Check sheet for the modelled part. Datum: model origin and axes. Units: mm. Face numbers are marked on the shaded views. A direction names the side the tool comes from. Coordinates: 2 decimals unless noted, no trailing zeros. Loops run counter-clockwise (first coordinate to the right, second up) from the corner with the lowest first, then second, coordinate; pieces in that order, holes last. Notation, with made-up numbers: M 49.5,35 L 80.5,35 A11 ccw 80.5,44 Z; hole C 83.5,47.5 d11. An arc over 180 degrees is marked long. Return JSON: item names as keys, results as strings.
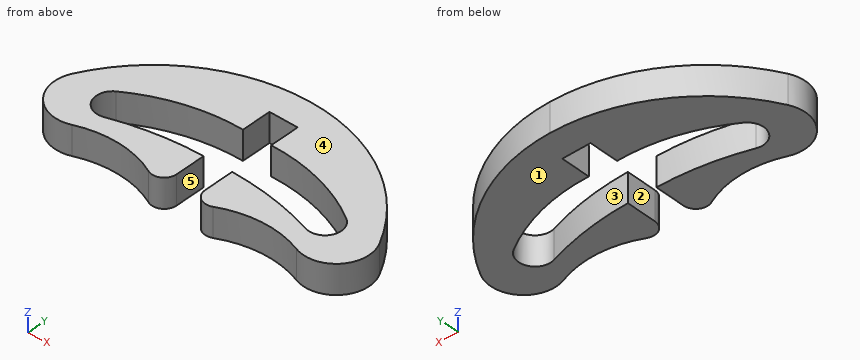
from build123d import *

# Parameters (mm, degrees)
EXTRUDE_1_DEPTH     = 3
SKETCH_2_W          = 2.925
SKETCH_2_H          = 8.058162309
CUT_EXTRUDE_1_DEPTH = 3
FILLET_1_R          = 1.27


with BuildPart() as part:
    # 스케치1 → 보스-돌출1 (new body)
    with BuildSketch(Plane.XY):
        with BuildLine():
            Line((-1.4475, 2.128), (-1.4475, 5.128))
            Line((-1.4475, 5.128), (1.4475, 5.128))
            Line((1.4475, 5.128), (1.4475, 2.128))
            ThreePointArc((1.4475, 2.128), (6.843352857, 1.44491364), (11.796869597, -0.801084345))
            ThreePointArc((11.796869597, -0.801084345), (12.394248626, -2.935784128), (10.351605925, -3.7968391))
            ThreePointArc((10.351605925, -3.7968391), (5.891355798, -2.693189603), (1.311601441, -2.322078509))
            Line((1.311601441, -2.322078509), (1.311601441, -7.845124291))
            ThreePointArc((1.311601441, -7.845124291), (6.16890602, -5.580674334), (11.498183086, -6.146313204))
            ThreePointArc((11.498183086, -6.146313204), (15.270849943, -5.260819217), (15.756720066, -1.416206748))
            ThreePointArc((15.756720066, -1.416206748), (9.210946066, 5.555889316), (0, 8.128))
            ThreePointArc((0, 8.128), (-9.210946066, 5.555889316), (-15.756720066, -1.416206748))
            ThreePointArc((-15.756720066, -1.416206748), (-15.270849943, -5.260819217), (-11.498183086, -6.146313204))
            ThreePointArc((-11.498183086, -6.146313204), (-6.16890602, -5.580674334), (-1.311601441, -7.845124291))
            Line((-1.311601441, -7.845124291), (-1.311601441, -2.322078509))
            ThreePointArc((-1.311601441, -2.322078509), (-5.891355798, -2.693189603), (-10.351605925, -3.7968391))
            ThreePointArc((-10.351605925, -3.7968391), (-12.394248626, -2.935784128), (-11.796869597, -0.801084345))
            ThreePointArc((-11.796869597, -0.801084345), (-6.843352857, 1.44491364), (-1.4475, 2.128))
        make_face()
    extrude(amount=EXTRUDE_1_DEPTH)

    # 스케치2 → 컷-돌출1 (cut)
    with BuildSketch(Plane.XY.offset(3)):
        with Locations((0, -5.233231355)):
            Rectangle(SKETCH_2_W, SKETCH_2_H)
    extrude(amount=-CUT_EXTRUDE_1_DEPTH, mode=Mode.SUBTRACT)

    # 필렛1
    fillet_1_edges = [part.edges().sort_by_distance(p)[0] for p in [
        (1.4625, -7.718694121, 1.5),
        (-1.4625, -7.718694121, 1.5),
    ]]
    fillet(fillet_1_edges, radius=FILLET_1_R)


solid = part.part
1) Draft check along X on the marked faces 4 and 5. Enter one of: +X half, -X half, draft (parallel to the pull), parting line (faces both ways), or undercut.
Answers:
{"face 4": "draft", "face 5": "undercut"}
2) Section check C-C on z = 1.2. Record the cut outline in (x, y).
Answers:
{"outline": "M -15.76,-1.42 A3.4 ccw -11.5,-6.15 A10.01 cw -3.3,-6.52 A1.27 ccw -1.46,-5.38 L -1.46,-2.32 A28.44 ccw -10.35,-3.8 A1.68 cw -11.8,-0.8 A18.21 cw -1.45,2.13 L -1.45,5.13 L 1.45,5.13 L 1.45,2.13 A18.21 cw 11.8,-0.8 A1.68 cw 10.35,-3.8 A28.44 ccw 1.46,-2.32 L 1.46,-5.38 A1.27 ccw 3.3,-6.52 A10.01 cw 11.5,-6.15 A3.4 ccw 15.76,-1.42 A17.78 ccw Z"}
3) Scan lines: line 1 along Y through (x, z) = (0.5, 1.8); line 2 along Y through (x, z) = (9, 1.85); line 3 along X through (y, z) = (-4.25, 2.5). Record each from-to range of solid material in increasing order. Write a range as [from, to].
Answers:
{"line 1": "[5.13, 8.12]", "line 2": "[-5.51, -3.38], [0.69, 5.68]", "line 3": "[-15.9, -1.46], [1.46, 15.9]"}
4) Set-up check for the marked faces 1, 2 and 3: record each of +Z, -Z, +X, -X, +Y, -Y from which the full face is reachable in a straight line by a thin tool's end or side.
Answers:
{"face 1": "-Z, +X, -X, +Y, -Y", "face 2": "+Z, -Z, -Y", "face 3": "+Z, -Z"}
5) Section check B-B on y = -4.75. Record the cut outline in (x, z), then the cut area to 3 significant figures.
Answers:
{"outline": "M -15.65,0 L -1.46,0 L -1.46,3 L -15.65,3 Z; M 1.46,0 L 15.65,0 L 15.65,3 L 1.46,3 Z", "area": "85.1 mm²"}
6) Section check A-A on x = -10. Record the cut outline in (y, z).
Answers:
{"outline": "M -5.69,0 L -3.68,0 L -3.68,3 L -5.69,3 Z; M 0.22,0 L 5.05,0 L 5.05,3 L 0.22,3 Z"}
7) Go/stop test with flat-tipped pins: pin 1 Ø0.9 at (y, z) = (-4, 1.5) entering from -X; pin 2 Ø1 at (y, z) = (-2, 1.5) entering from +X; pin 3 Ø0.9 at (y, z) = (4, 1.5) entering from -X. Record where each tip stops, or that it passes through.
Answers:
{"pin 1": "x = -16.1", "pin 2": "x = 16.11", "pin 3": "x = -11.91"}
8) Section check D-D on x = 14. Record the cut outline in (y, z).
Answers:
{"outline": "M -6.14,0 L 1.31,0 L 1.31,3 L -6.14,3 Z"}
